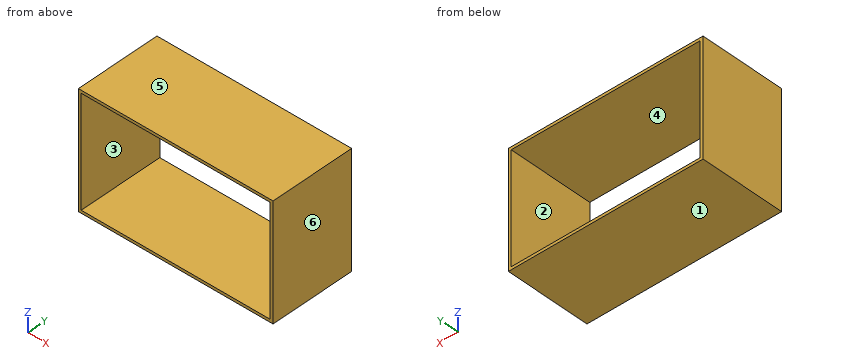
```python
from build123d import *

# Parameters (mm, degrees)
F0_W     = 1100
F0_H     = 650
F1_DEPTH = 478


with BuildPart() as f1:
    # F0 (on Front) → F1 (new body)
    with BuildSketch(Plane.XZ):
        Rectangle(F0_W, F0_H)
        Polygon((-534, 103), (-534, 309), (-234, 309), (-218, 309), (-202, 309), (202, 309), (218, 309), (234, 309), (534, 309), (534, 103), (534, -103), (534, -309), (234, -309), (218, -309), (202, -309), (-202, -309), (-218, -309), (-234, -309), (-534, -309), (-534, -103), align=None, mode=Mode.SUBTRACT)
    extrude(amount=-F1_DEPTH)


solid = f1.part
```
Read the model definition and answer for the solid it produces. Units are mm, in the model's axes. Face numbers are marked on the shaded views. A direction names the side the tool comes from. Give positions to 0.01 mm unless a question says otherwise; leave off trailing zeros. Order: outer loops, then holes, each group sorted by start corner. A loop starts at its lowest first (then second) coordinate and runs counter-clockwise, first axis right, second up. Notation, with made-up numbers: (-10, -23) -> (38, -23) arc R33 cw to (38, 6) -> close; hole circle Ø11 at (-39.5, -23.5). An arc over 180 degrees is marked (long way). One line per item, written item: value. Start each with the question number.
(1) A tool of negligible diameter and unlimited length cuts with its end or side. For the marked faces 1 and 2, from which of +Z, -Z, +X, -X, +Y, -Y can it reach the whole face along a straight path? Write none if from no direction.
(2) The part is cut by section A-A (z = -261). Determine the outline of the cut face in (x, y), and give its area (3 significant figures).
(3) Straight lines are drawn through the part: L1, parallel to X at y = 68.5, z = 237.5; L2, parallel to Z at x = -109, y = 349.5. For each, find the intervals that lie inside material, in ascending order.
(4) The part is cut by section B-B (y = 256.5). Determine the outline of the cut face in (x, z).
(5) For a pull along X with two mould halves and no side action, classify the marked faces 3, 4, 5 and 6 as released by +X, released by -X, zero draft, split by the parting line, or undercut.
(6) The part is cut by section C-C (x = -448.5). Determine the outline of the cut face in (y, z), and give its area (3 significant figures).
Taken from the geometry:
1. face 1: -Z, +X, -X, +Y, -Y
1. face 2: +Y, -Y
2. outline: (-550, 0) -> (-534, 0) -> (-534, 478) -> (-550, 478) -> close; (534, 0) -> (550, 0) -> (550, 478) -> (534, 478) -> close
2. area: 15,300 mm^2
3. L1: -550 to -534, 534 to 550
3. L2: -325 to -309, 309 to 325
4. outline: (-550, -325) -> (550, -325) -> (550, 325) -> (-550, 325) -> close; hole (-534, -309) -> (534, -309) -> (534, 309) -> (-534, 309) -> close
5. face 3: undercut
5. face 4: undercut
5. face 5: zero draft
5. face 6: released by +X
6. outline: (0, -325) -> (478, -325) -> (478, -309) -> (0, -309) -> close; (0, 309) -> (478, 309) -> (478, 325) -> (0, 325) -> close
6. area: 15,300 mm^2
